Can you work these out from the model? Positions are in its coordinate system, mm. A direction names the side the tool comes from. Coordinates: 2 decimals unless noted, no trailing zeros. Write each loop counter-clockwise with the first axis right and the second up, starting at its lowest first coordinate (ties: lowest second). Pieces come first, ordered by that corner, then holes. Notation, with made-up numbers: (5.5, 77.5) - (60.5, 77.5) arc R16 ccw to (60.5, 108.5) - close; hole circle Ø9 at (29.5, 37). An arc over 180 degrees is marked (long way). Use one line per item in the form item = value. Start each with the question number.
(1) On a 3-axis mill with a long thin cutter (end or side, diameter ignored), from which of +Z, -Z, +X, -X, +Y, -Y can I reach the whole of each face in a straight line? I mean faces 1 (the face through (49.558, -50, 65)), 2 (the face through (17, -50, 32.144)), 3 (the face through (56, -30.388, 15)), 4 (the face through (12, -58, 50.316)), 5 (the face through (51, -15, 30.48)). Say none if no direction works.
(2) If we section it at A-A on y = -63: Please give me the cut outline in (x, z).
(3) If we section it at B-B on x = 10.5: Please give me the cut outline in (y, z).
(4) If we section it at D-D on y = -39: Please give me the cut outline in (x, z).
(5) For pin 1 Ø9 at (x, y) = (55, -17) entering from -Z; pin 2 Ø4 at (y, z) = (-51.5, 62) entering from -X; pin 3 Ø20 at (x, y) = (6.5, -65) entering from +Z; pin 4 Ø8 at (x, z) = (26.5, 30) entering from -Y, each with a flat end and sliding along its axis, tell me the tip position at first contact or that it passes through.
(6) If we section it at C-C on z = 11.5: Please give me the cut outline in (x, y), then the cut area to 3 significant figures.
(7) If I drill on probe 1 along Z at (x, y) = (15, -70.5); probe 2 along Y at (x, z) = (71, 62); probe 3 along Y at (x, z) = (71.5, 18), over which ranges is the centre line in solid material (lowest first)? Write a range as from..to.
```python
from build123d import *

# Parameters (mm, degrees)
F0_W      = 75.7038891315
F0_H      = 75.1095712185
F1_DEPTH  = 76.1847347021
F3_DEPTH  = 7.5595728122
F4_W      = 75.7038891315
F4_H      = 76.1847347021
F5_DEPTH  = 70.3715533018
F6_W      = 35.1695269346
F6_H      = 32.1441143751
F7_DEPTH  = 50.8
F8_W      = 26.1460281909
F8_H      = 21.5719044209
F9_DEPTH  = 50.8
F10_W     = 30.3881298751
F10_H     = 30.4796360433
F11_DEPTH = 50.8
F13_W     = 25.1194015145
F13_H     = 34.0582877398
F14_DEPTH = 25.8685164154


with BuildPart() as f1:
    # F0 (on Top) → F1 (new body)
    with BuildSketch(Plane.XY):
        with Locations((37.8519445658, -37.5547856092)):
            Rectangle(F0_W, F0_H)
    extrude(amount=F1_DEPTH)

    # F2 (on face) → F3 (join)
    with BuildSketch(Plane.XZ.offset(75.1095712185)):
        Polygon((75.7038891315, 0), (38.7951347365, 39.0415483477), (0, 0), align=None)
        Polygon((75.7038891315, 76.1847347021), (37.8519445658, 40.0392413139), (38.7951347365, 39.0415483477), align=None)
        Polygon((75.7038891315, 76.1847347021), (0, 76.1847347021), (37.8519445658, 40.0392413139), align=None)
    extrude(amount=-F3_DEPTH)

    # F4 (on face) → F5 (join)
    with BuildSketch(Plane.XZ.offset(75.1095712185)):
        with Locations((37.8519445658, 38.0923673511)):
            Rectangle(F4_W, F4_H)
    extrude(amount=-F5_DEPTH)

    # F6 (on face) → F7 (cut)
    with BuildSketch(Plane.XZ.offset(75.1095712185)):
        with Locations((17.5847634673, 16.0720571876)):
            Rectangle(F6_W, F6_H)
    extrude(amount=-F7_DEPTH, mode=Mode.SUBTRACT)

    # F8 (on face) → F9 (cut)
    with BuildSketch(Plane.XZ.offset(75.1095712185)):
        with Locations((62.6308750361, 65.3987824917)):
            Rectangle(F8_W, F8_H)
    extrude(amount=-F9_DEPTH, mode=Mode.SUBTRACT)

    # F10 (on face) → F11 (cut)
    with BuildSketch(Plane.YZ.offset(75.7038891315)):
        with Locations((-15.1940649375, 15.2398180217)):
            Rectangle(F10_W, F10_H)
    extrude(amount=-F11_DEPTH, mode=Mode.SUBTRACT)

    # F13 (on face) → F14 (cut)
    with BuildSketch(Plane.XY.offset(76.1847347021)):
        with Locations((12.5597007573, -58.0804273486)):
            Rectangle(F13_W, F13_H)
    extrude(amount=-F14_DEPTH, mode=Mode.SUBTRACT)


solid = f1.part
```
Reported:
q1.face_1 = +Z, +X, -Y
q1.face_2 = -Z, -X, -Y
q1.face_3 = -Z, +X, -X, +Y
q1.face_4 = +Z, -X, -Y
q1.face_5 = -Z, +X, +Y
q2.outline = (0, 32.14) - (35.17, 32.14) - (35.17, 0) - (75.7, 0) - (75.7, 54.61) - (49.56, 54.61) - (49.56, 76.18) - (25.12, 76.18) - (25.12, 50.32) - (0, 50.32) - close
q3.outline = (-75.11, 32.14) - (-24.31, 32.14) - (-24.31, 0) - (0, 0) - (0, 76.18) - (-41.05, 76.18) - (-41.05, 50.32) - (-75.11, 50.32) - close
q4.outline = (0, 32.14) - (35.17, 32.14) - (35.17, 0) - (75.7, 0) - (75.7, 54.61) - (49.56, 54.61) - (49.56, 76.18) - (0, 76.18) - close
q5.pin_1 = 30.48
q5.pin_2 = 25.12
q5.pin_3 = 50.32
q5.pin_4 = -75.11
q6.outline = (0, -24.31) - (24.9, -24.31) - (24.9, 0) - (0, 0) - close; (35.17, -75.11) - (75.7, -75.11) - (75.7, -30.39) - (35.17, -30.39) - close
q6.area = 2,420 mm2
q7.probe_1 = 32.14..50.32
q7.probe_2 = -24.31..0
q7.probe_3 = -75.11..-30.39
